Autodesk Inventor part; units mm, degrees
ref_plane "YZ Plane" through (0, 0, 0) normal (1, 0, 0) x (0, 1, 0)
ref_plane "XZ Plane" through (0, 0, 0) normal (0, 1, 0) x (-1, 0, 0)
ref_plane "XY Plane" through (0, 0, 0) normal (0, 0, 1) x (1, 0, 0)
sketch "Sketch5" plane through (0, 0, 0) normal (0, 1, 0) x (-1, 0, 0)
  circle A0 centre (0, 0) radius 1.75
  circle A1 centre (0, 0) radius 40
  line L0 (0, 0) -> (40, 0)
  line L1 (40, 0) -> (45, 0)
  line L2 (40, 0) -> (40, -5)
  line L3 (40, 0) -> (45, 0) construction
  line L4 (40, -5) -> (0, -5)
  line L5 (0, -5) -> (0, 5)
  line L6 (0, 5) -> (40, 5)
  line L7 (40, 5) -> (40, -5)
  line L8 (-15.6699, 37.141) -> (4.3301, 2.5)
  line L9 (-4.3301, -2.5) -> (-24.3301, 32.141)
  line L10 (4.3301, 2.5) -> (-4.3301, -2.5)
  line L11 (-20, 34.641) -> (-15.6699, 37.141)
  line L12 (-24.3301, 32.141) -> (-15.6699, 37.141)
  line L13 (-24.3301, -32.141) -> (-4.3301, 2.5)
  line L14 (4.3301, -2.5) -> (-15.6699, -37.141)
  line L15 (-4.3301, 2.5) -> (4.3301, -2.5)
  line L16 (-20, -34.641) -> (-24.3301, -32.141)
  line L17 (-15.6699, -37.141) -> (-24.3301, -32.141)
  dimension "d78" = 80
  dimension "d54" = 3.5
  dimension "d82" = 5
  dimension "d83" = 5
  dimension "d84" = 90
  dimension "d85" = 40
  dimension "d86" = 10
  dimension "d89" = 360
extrude "Extrusion7" add sketch "Sketch5" along normal blind 10 contours L0 L10 A0 | L0 A1 L4 L14 L15 A0 | A0 L15 L0 | A0 L10 L8 L6 A1 L0 | L10 L5 A0 | A0 L5 L6 L8 L10 | L15 L14 L4 L5 A0 | A0 L5 L15 | L15 A0 L5 | L5 A0 L10 | L10 A0 L15 | L2 L4 A1 | A1 L6 L7 | A0 L15 L13 L9 A1 L8 L6 L5 | L5 L4 L14 A1 L13 L9 L10 A0 | L10 L9 L13 L15 A0 | A1 L11 L8 | L14 L17 A1 | A1 L9 L12 | L16 L13 A1
sketch "Sketch7" plane through (5.7735, 0, 0) normal (0.866, 0, 0.5) x (0.5, 0, -0.866)
  line L0 (37.1132, 0) -> (37.1132, 10)
  line L1 (37.1132, 10) -> (37.1132, 5)
  line L2 (37.1132, 5) -> (32.1132, 5)
  circle A0 centre (32.1132, 5) radius 1.5
  point P0 (-2.8868, 0)
  dimension "d93" = 5
  dimension "d94" = 5
  dimension "d95" = 3
extrude "Extrusion8" cut sketch "Sketch7" against normal blind 20
sketch "Sketch8" plane through (0, 10, 0) normal (0, 1, 0) x (1, 0, 0)
  circle A0 centre (0, 0) radius 1.75
  dimension "d98" = 3.5
extrude "Extrusion9" cut sketch "Sketch8" against normal blind 10
pattern_circular "Circular Pattern7" count 3 over 360 about axis through (0, 10, 0) along (0, -1, 0) of "Extrusion8"
fillet "Fillet7" radius 10 3 edges at (5.7735, 5, 0) (-2.8868, 5, 5) (-2.8868, 5, -5)
fillet "Fillet8" radius 2 23 edges at (15.6699, 5, 37.141) (24.3301, 5, 32.141) (-40, 5, 5) (-40, 10, 0) (24.3301, 5, -32.141) (20, 10, -34.641) (15.6699, 5, -37.141) (-24.3301, 10, -5) (7.8349, 10, -23.5705) (16.4952, 10, 18.5705) (16.4952, 10, -18.5705) (-24.3301, 10, 5) (7.8349, 10, 23.5705) (-40, 5, -5) (-40, 0, 0) (20, 0, 34.641) (16.4952, 0, -18.5705) (16.4952, 0, 18.5705) (-24.3301, 0, 5) (7.8349, 0, 23.5705) (-24.3301, 0, -5) (7.8349, 0, -23.5705) (20, 0, -34.641)
properties part number "Custom_Delta_End_Effector"
The listing builds one solid part. Answer for the finished solid, in the listing's coordinates (mm). A direction names the side the tool comes from. Round coordinates to 2 decimals unless told otherwise and drop trailing zeros. Write each loop counter-clockwise with the first axis right and the second up, starting at its lowest first coordinate (ties: lowest second). Pieces come first, ordered by that corner, then holes. Notation, with made-up numbers: M 81.5,3 L 89.5,3 A20 ccw 89.5,15 Z; hole C 53,36.25 d2. An arc over 180 degrees is marked long. Write each question's results on one line, items separated by ' | '. Start each with the question number.
Item 1: For faces 1 (the face through (15.577, 9.43, -18.183)), 2 (the face through (15.577, 0.57, 18.183)), 3 (the face through (-23.54, 9.4, 4.43)), 4 (the face through (-23.12, 9.4, -4.43)), determine the directions among +Z, -Z, +X, -X, +Y, -Y from which every point of the face is accessible in a straight line to the end or side of a thin tool.
Item 2: A cutting plane is placed at C-C on y = 9. Write down the section's boundary in (x, z).
Item 3: For a pull along Z with two mould halves and no side action, classify faces 5 (the face through (-39.4, 5.04, -4.43)), 6 (the face through (15.863, 6.056, 36.335)), 7 (the face through (7.32, 5.04, -0.07)) as pulls with the +Z half, pulls with the -Z half, needs draft (parallel to the pull), parting line crosses it, or undercut.
Item 4: Straight lines are drawn through the part: L1, parallel to X at y = 7, z = 0; L2, parallel to Z at x = 0, y = 5.75; L3, parallel to Z at x = -15, y = 5.25. For each, find the intervals that lie inside material, in ascending order. Write a range as [from, to].
Item 5: Flat-ended cylindrical pins translate along their axes: pin 1 Ø1.8 at (x, y) = (-19.5, 6) entering from -Z; pin 2 Ø1 at (x, y) = (15, 7.5) entering from -Z; pin 3 Ø1 at (x, y) = (17, 6.5) entering from +Z; pin 4 Ø3 at (x, z) = (0, 0) entering from -Y. Find the tip coordinate at first contact, or state that the pin passes through.
Item 6: A cutting plane is placed at B-B on x = -15.5. Write down the section's boundary in (y, z), and give its area (3 significant figures).
Item 7: A cutting plane is placed at A-A on z = 0. Write down the section's boundary in (x, y).
Check sheet entries:
1) face 1: +X, +Y | face 2: +X, -Y | face 3: +Z, -X, +Y | face 4: -Z, -X, +Y
2) outline: M -39.73,-3 A1.73 ccw -38,-4.73 L -8.66,-4.73 A10.27 cw 0.23,-9.87 L 14.9,-35.27 A1.73 ccw 17.27,-35.91 L 22.46,-32.91 A1.73 ccw 23.1,-30.54 L 8.43,-5.13 A10.27 cw 8.43,5.13 L 23.6,31.41 A2 ccw 22.6,33.14 L 17.4,36.14 A2 ccw 15.4,36.14 L 0.23,9.87 A10.27 cw -8.66,4.73 L -38,4.73 A1.73 ccw -39.73,3 Z; hole C 0,0 d3.5
3) face 5: pulls with the -Z half | face 6: pulls with the +Z half | face 7: undercut
4) L1: [-40, -1.75], [1.75, 7.32] | L2: [-10, -1.75], [1.75, 10] | L3: [-5, 5]
5) pin 1: z = -5 | pin 2: z = -36.19 | pin 3: z = 36.41 | pin 4: through
6) outline: M 0,-3 A2 ccw 2,-5 L 8,-5 A2 ccw 10,-3 L 10,3 A2 ccw 8,5 L 2,5 A2 ccw 0,3 Z | area: 96.6 mm²
7) outline: M -40,2 A2 ccw -38,0 L -1.75,0 L -1.75,10 L -38,10 A2 ccw -40,8 Z; M 1.75,0 L 5.32,0 A2 ccw 7.32,2 L 7.32,8 A2 ccw 5.32,10 L 1.75,10 Z; hole C -35,5 d3
